Could you check a few things on this drawing? It's one solid part, dimensions in mm from its lowest x, y, z. A direction names the side the tool comes from. Round coordinates to 2 decimals unless told otherwise and drop trailing zeros. Write each loop counter-clockwise with the first axis right and the second up, starting at its lowest first coordinate (ties: lowest second). Pieces come first, ordered by that corner, then holes. Notation, with made-up numbers: (-31.75, -37) -> (16.25, -37) arc R11 cw to (16.25, -21) -> close; hole circle Ø1 at (21.25, -3). An arc over 180 degrees is marked (long way). Put each result on its own line as item: value. Start each with the question number.
1) I want a section at A-A, the plane z = 10. List the corners of the cut face in (x, y) for me.
2) If I drill on line 1 along Z through (x, y) = (1.1, 18.8); line 2 along Y through (x, z) = (17.5, 1.75); line 3 along Y through (x, z) = (1.05, 14.75), over which ranges is the centre line in solid material (lowest first)? Write a range as [from, to].
3) Will these pins go through, and if not, where does the flat tip stop? P1, Ø6, axis at x = 13, z = 8.5, coming from the +Y side; P2, Ø3, axis at y = 4, z = 12, coming from the +X side.
4) I want a section at D-D, the plane z = 5.25. List the corners of the cut face in (x, y) for me, then the cut area to 3 significant figures.
5) I want a section at B-B, the plane y = 18.8. List the corners of the cut face in (x, z) for me.
6) Which directions (+Z, -Z, +X, -X, +Y, -Y) give clear straight access to the entire face, cutting with the end or side of a thin tool? Please do the marked faces 1 and 2.
7) I want a section at C-C, the plane x = 15.5. List the corners of the cut face in (y, z) for me.
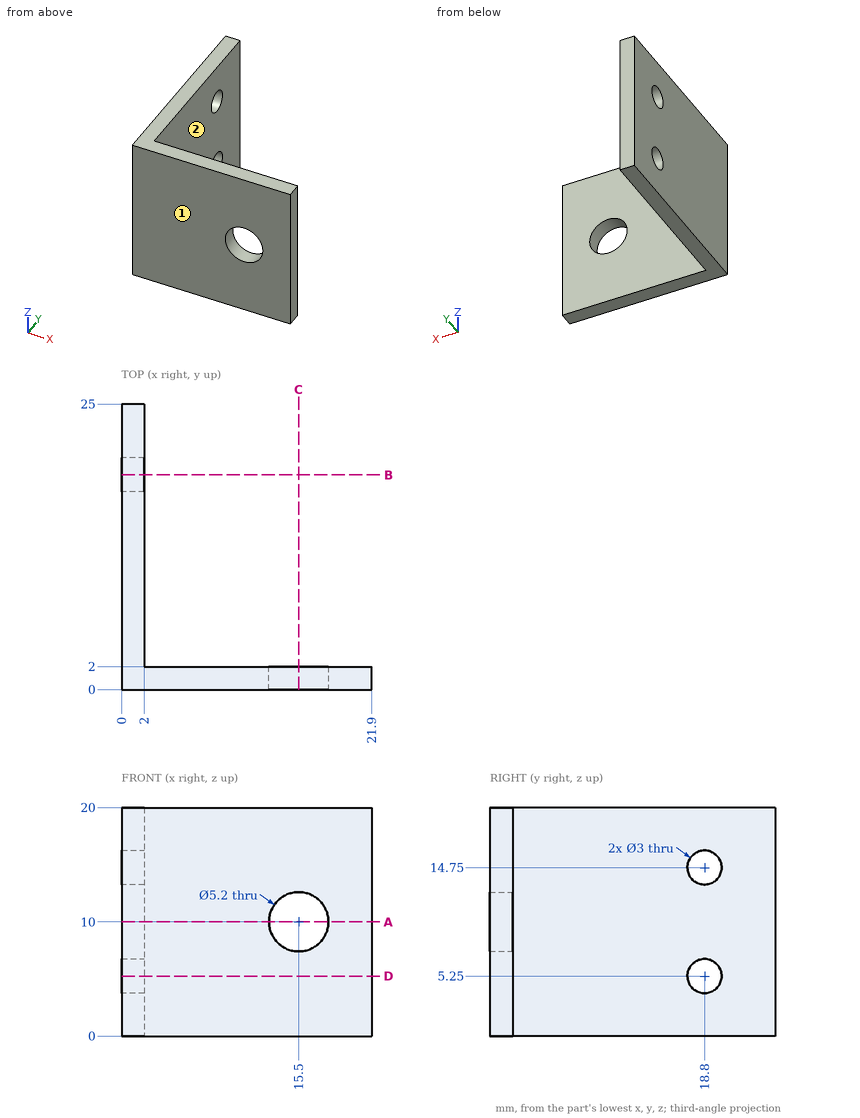
Findings:
1. outline: (0, 0) -> (12.9, 0) -> (12.9, 2) -> (2, 2) -> (2, 25) -> (0, 25) -> close; (18.1, 0) -> (21.9, 0) -> (21.9, 2) -> (18.1, 2) -> close
2. line 1: z = [0, 3.75], [6.75, 13.25], [16.25, 20]
2. line 2: y = [0, 2]
2. line 3: y = [0, 17.3], [20.3, 25]
3. P1: stops at y = 2
3. P2: stops at x = 2
4. outline: (0, 0) -> (21.9, 0) -> (21.9, 2) -> (2, 2) -> (2, 17.3) -> (0, 17.3) -> close; (0, 20.3) -> (2, 20.3) -> (2, 25) -> (0, 25) -> close
4. area: 83.8 mm2
5. outline: (0, 0) -> (2, 0) -> (2, 3.75) -> (0, 3.75) -> close; (0, 6.75) -> (2, 6.75) -> (2, 13.25) -> (0, 13.25) -> close; (0, 16.25) -> (2, 16.25) -> (2, 20) -> (0, 20) -> close
6. face 1: +Z, -Z, +X, -X, -Y
6. face 2: +Z, -Z, +X, +Y
7. outline: (0, 0) -> (2, 0) -> (2, 7.4) -> (0, 7.4) -> close; (0, 12.6) -> (2, 12.6) -> (2, 20) -> (0, 20) -> close
